```python
from build123d import *

# Parameters (mm, degrees)
SKETCH1_W           = 36.526911934
SKETCH1_H           = 36.526911934
BOSS_EXTRUDE1_DEPTH = 5
CAVITY1_START       = -2
CAVITY1_DEPTH       = 2


with BuildPart() as part:
    # Sketch1 → Boss-Extrude1 (new body)
    with BuildSketch(Plane.XY):
        Rectangle(SKETCH1_W, SKETCH1_H)
    extrude(amount=-BOSS_EXTRUDE1_DEPTH)

    # Cavity1: read off the stored shape, not the designer's step
    # Cavity1 outline → Cavity1 (cut)
    with BuildSketch(Plane.XY.offset(CAVITY1_START)):
        with BuildLine():
            Line((16.263455967, -12.263455967), (16.263455967, 12.263455967))
            ThreePointArc((16.263455967, 12.263455967), (15.091883092, 15.091883092), (12.263455967, 16.263455967))
            Line((12.263455967, 16.263455967), (-12.263455967, 16.263455967))
            ThreePointArc((-12.263455967, 16.263455967), (-15.091883092, 15.091883092), (-16.263455967, 12.263455967))
            Line((-16.263455967, 12.263455967), (-16.263455967, -12.263455967))
            ThreePointArc((-16.263455967, -12.263455967), (-15.091883092, -15.091883092), (-12.263455967, -16.263455967))
            Line((-12.263455967, -16.263455967), (12.263455967, -16.263455967))
            ThreePointArc((12.263455967, -16.263455967), (15.091883092, -15.091883092), (16.263455967, -12.263455967))
        make_face()
    extrude(amount=CAVITY1_DEPTH, mode=Mode.SUBTRACT)

    # Cavity1 2: loft between two sections, ruled curve by curve
    cavity1_2_from = [
        Edge.make_three_point_arc((14.263455967, 12.263455967, -4), (13.67766953, 13.67766953, -4), (12.263455967, 14.263455967, -4)),
        Edge.make_three_point_arc((-12.263455967, 14.263455967, -4), (-13.67766953, 13.67766953, -4), (-14.263455967, 12.263455967, -4)),
        Edge.make_three_point_arc((12.263455967, -14.263455967, -4), (13.67766953, -13.67766953, -4), (14.263455967, -12.263455967, -4)),
        Edge.make_three_point_arc((-14.263455967, -12.263455967, -4), (-13.67766953, -13.67766953, -4), (-12.263455967, -14.263455967, -4)),
        Edge.make_line((-12.263455967, 14.263455967, -4), (12.263455967, 14.263455967, -4)),
        Edge.make_line((14.263455967, 12.263455967, -4), (14.263455967, -12.263455967, -4)),
        Edge.make_line((-14.263455967, 12.263455967, -4), (-14.263455967, -12.263455967, -4)),
        Edge.make_line((12.263455967, -14.263455967, -4), (-12.263455967, -14.263455967, -4)),
    ]
    cavity1_2_to = [
        Edge.make_three_point_arc((16.263455967, 12.263455967, -2), (15.091883092, 15.091883092, -2), (12.263455967, 16.263455967, -2)),
        Edge.make_three_point_arc((-12.263455967, 16.263455967, -2), (-15.091883092, 15.091883092, -2), (-16.263455967, 12.263455967, -2)),
        Edge.make_three_point_arc((12.263455967, -16.263455967, -2), (15.091883092, -15.091883092, -2), (16.263455967, -12.263455967, -2)),
        Edge.make_three_point_arc((-16.263455967, -12.263455967, -2), (-15.091883092, -15.091883092, -2), (-12.263455967, -16.263455967, -2)),
        Edge.make_line((-12.263455967, 16.263455967, -2), (12.263455967, 16.263455967, -2)),
        Edge.make_line((16.263455967, 12.263455967, -2), (16.263455967, -12.263455967, -2)),
        Edge.make_line((-16.263455967, 12.263455967, -2), (-16.263455967, -12.263455967, -2)),
        Edge.make_line((12.263455967, -16.263455967, -2), (-12.263455967, -16.263455967, -2)),
    ]
    cavity1_2 = Solid(Shell([*[Face.make_surface_from_curves(cavity1_2_from[k], cavity1_2_to[k]) for k in range(8)], Face(Wire(cavity1_2_from)), Face(Wire(cavity1_2_to))]))
    add(cavity1_2, mode=Mode.SUBTRACT)


solid = part.part
```
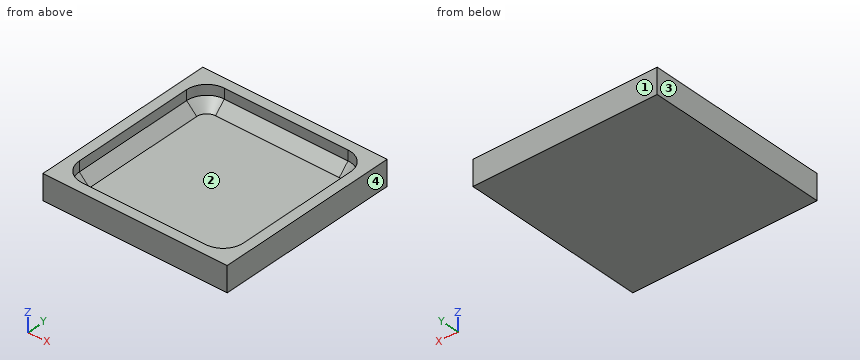
Read the model definition and answer for the solid it produces. Units are mm, in the model's axes. Face numbers are marked on the shaded views. Coordinates: 2 decimals unless noted, no trailing zeros. Write each loop counter-clockwise with the first axis right and the second up, starting at its lowest first coordinate (ties: lowest second). Pieces come first, ordered by that corner, then holes. Notation, with made-up numbers: (-23, -29.5) -> (12, -29.5) arc R33 cw to (12, 2.5) -> close; hole circle Ø3 at (72.25, 34). An arc over 180 degrees is marked (long way). Answer as a JSON object with one key per item and string values.
Q1. Determine the mould class of the marked faces 1, 2, 3 and 4 for opening direction X: pulls with the +X half, pulls with the -X half, needs draft (parallel to the pull), parting line crosses it, or undercut.
The answers:
{"face 1": "needs draft", "face 2": "undercut", "face 3": "pulls with the -X half", "face 4": "pulls with the +X half"}
Q2. A flat-ended cylindrical pin translates along its axis: pin 1 Ø14.5 at (x, y) = (-5.5, 0.5) entering from +Z. Find the tip coordinate at first contact, or state that the pin passes through.
The answers:
{"pin 1": "stops at z = -4"}
Q3. The part is cut by section A-A on z = -0.9. Give the vertices of the cut face in (x, y), then the cut area to 3 significant figures.
The answers:
{"outline": "(-18.26, -18.26) -> (18.26, -18.26) -> (18.26, 18.26) -> (-18.26, 18.26) -> close; hole (-16.26, -12.26) arc R4 ccw to (-12.26, -16.26) -> (12.26, -16.26) arc R4 ccw to (16.26, -12.26) -> (16.26, 12.26) arc R4 ccw to (12.26, 16.26) -> (-12.26, 16.26) arc R4 ccw to (-16.26, 12.26) -> close", "area": "290 mm2"}
Q4. Consider line 1 (Y direction, x = -1, z = -2); line 2 (Z direction, x = 7.5, y = -4). Determine where each line is inside the solid, lowest interval first. Write a range as [from, to].
The answers:
{"line 1": "y = [-18.26, -16.26], [16.26, 18.26]", "line 2": "z = [-5, -4]"}
